For this review, take the finished solid that the model builds, in its own axes (mm). Face numbers are marked on the shaded views. Give positions to 0.01 mm unless a question says otherwise; leave off trailing zeros. Write each loop counter-clockwise with the first axis right and the second up, starting at its lowest first coordinate (ties: lowest second). Pieces come first, ordered by that corner, then holes.
Q1. For line 1 (Z direction, x = -26, y = -1.5); line 2 (Z direction, x = -15.5, y = -0.5); line 3 (Y direction, x = -7.5, z = 31.5), list the stretches that pass through material, from the lowest coordinate up.
Q2. Insertion check: P1, Ø5, axis at y = -4, z = 4.5, coming from the +X side; P2, Ø3, axis at y = -2, z = -18.5, coming from the -X side; P3, Ø1.5, axis at y = -8, z = 3, coming from the -X side. Each pin has a flat end and moves straight along its axis. Give the tip position at first contact, or say it passes through.
Q3. We need section C-C (y = -1.5). Write out the cut boundary in (x, z), then the cut area to 3 significant figures.
Q4. We need section B-B (z = -22). Write out the cut boundary in (x, y), then the cut area to 3 significant figures.
Q5. Mouldability with a two-part tool opening along X and no side actions: class the marked faces 1, 2, 3 and 4 as released by +X, released by -X, zero draft, split by the parting line, or undercut.
Q6. We need section D-D (x = 13). Write out the cut boundary in (y, z).
Q7. We need section A-A (x = 26). Write out the cut boundary in (y, z), then the cut area to 3 significant figures.
```python
from build123d import *

# Parameters (mm, degrees)
F1_DEPTH = 12.7
F2_SIZE  = 5.08
F3_T     = -2.54
F4_SIZE  = 5.08
F5_SIZE  = 5.08
F6_SIZE  = 5.08


# Not quite as in the source:
# - a feature of the source that left no trace in its solid (it failed there, or was rolled back) is left out


with BuildPart() as f1:
    # F0 (on Front) → F1 (new body)
    with BuildSketch(Plane.XZ):
        Polygon((0, 0), (-38.1, 38.1), (0, -38.1), align=None)
        Polygon((38.1, 38.1), (-38.1, 38.1), (0, 0), align=None)
        Polygon((0, 0), (0, -38.1), (38.1, 38.1), align=None)
    extrude(amount=F1_DEPTH)

    # F2
    f2_edges = [f1.edges().sort_by_distance(p)[0] for p in [
        (0, -12.7, 38.1),
        (-19.05, -12.7, 0),
        (19.05, -12.7, 0),
        (-19.05, 0, 0),
        (0, 0, 38.1),
        (19.05, 0, 0),
    ]]
    chamfer(f2_edges, length=F2_SIZE)

    # F3
    f3_openings = [f1.faces().sort_by_distance(p)[0] for p in [
        (0, 0, 13.099742),
    ]]
    offset(amount=F3_T, openings=f3_openings, kind=Kind.INTERSECTION)

    # F4
    f4_edges = [f1.edges().sort_by_distance(p)[0] for p in [
        (0, -12.7, 33.02),
        (14.940194, -12.7, 3.139613),
        (-14.940194, -12.7, 3.139613),
    ]]
    chamfer(f4_edges, length=F4_SIZE)

    # F5
    f5_edges = [f1.edges().sort_by_distance(p)[0] for p in [
        (0, -12.7, 27.94),
        (10.830387, -12.7, 6.279225),
        (-10.830387, -12.7, 6.279225),
    ]]
    chamfer(f5_edges, length=F5_SIZE)

    # F6
    f6_edges = [f1.edges().sort_by_distance(p)[0] for p in [
        (0, -12.7, 22.86),
        (6.720581, -12.7, 9.418838),
        (-6.720581, -12.7, 9.418838),
    ]]
    chamfer(f6_edges, length=F6_SIZE)


solid = f1.part
```
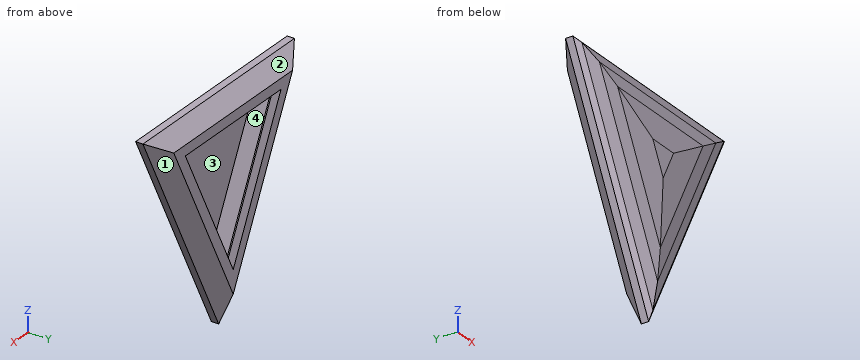
Computed:
1. line 1: z = 21.91 to 29.94, 30.93 to 34.52
1. line 2: z = 3.14 to 11.17, 29.93 to 33.52
1. line 3: y = -10.98 to -10.16, -2.07 to 0
2. P1: stops at x = 22.43
2. P2: stops at x = -8.19
2. P3: stops at x = -20.87
3. outline: (-32.31, 34.52) - (0, -30.09) - (32.31, 34.52) - close; hole (-26.5, 30.93) - (0, -22.06) - (26.5, 30.93) - close
3. area: 684 mm2
4. outline: (-8.05, -7.62) - (-6.39, -9.11) - (-1.94, -10.76) - (0, -11.1) - (1.94, -10.76) - (6.39, -9.11) - (8.05, -7.62) - (8.05, -5.08) - (2.37, 0) - (-2.37, 0) - (-8.05, -5.08) - close; hole (-5.21, -6.57) - (-1.19, -10.16) - (1.19, -10.16) - (5.21, -6.57) - (5.21, -6.13) - (0, -1.47) - (-5.21, -6.13) - close
4. area: 77.9 mm2
5. face 1: released by +X
5. face 2: zero draft
5. face 3: undercut
5. face 4: undercut
6. outline: (-12.23, 22.59) - (-11.71, 10.84) - (-10.76, 0.12) - (-9.11, -8.77) - (-7.62, -12.1) - (-5.08, -12.1) - (0, -0.74) - (0, 7.29) - (-6.13, -6.42) - (-6.57, -6.42) - (-10.16, 1.61) - (-10.16, 31.97) - (-6.57, 35.56) - (-6.13, 35.56) - (0, 29.43) - (0, 33.02) - (-5.08, 38.1) - (-7.62, 38.1) - (-9.11, 36.61) - (-10.76, 32.63) - (-11.71, 27.84) - close
7. outline: (-11.16, 30.62) - (-10.76, 26.12) - (-9.11, 17.23) - (-7.62, 13.9) - (-5.08, 13.9) - (0, 25.26) - (0, 33.02) - (-5.08, 38.1) - (-7.62, 38.1) - (-9.11, 36.61) - (-10.76, 32.63) - close; hole (-10.16, 27.61) - (-6.57, 19.58) - (-6.13, 19.58) - (-1.19, 30.62) - (-6.13, 35.56) - (-6.57, 35.56) - (-10.16, 31.97) - close
7. area: 115 mm2
